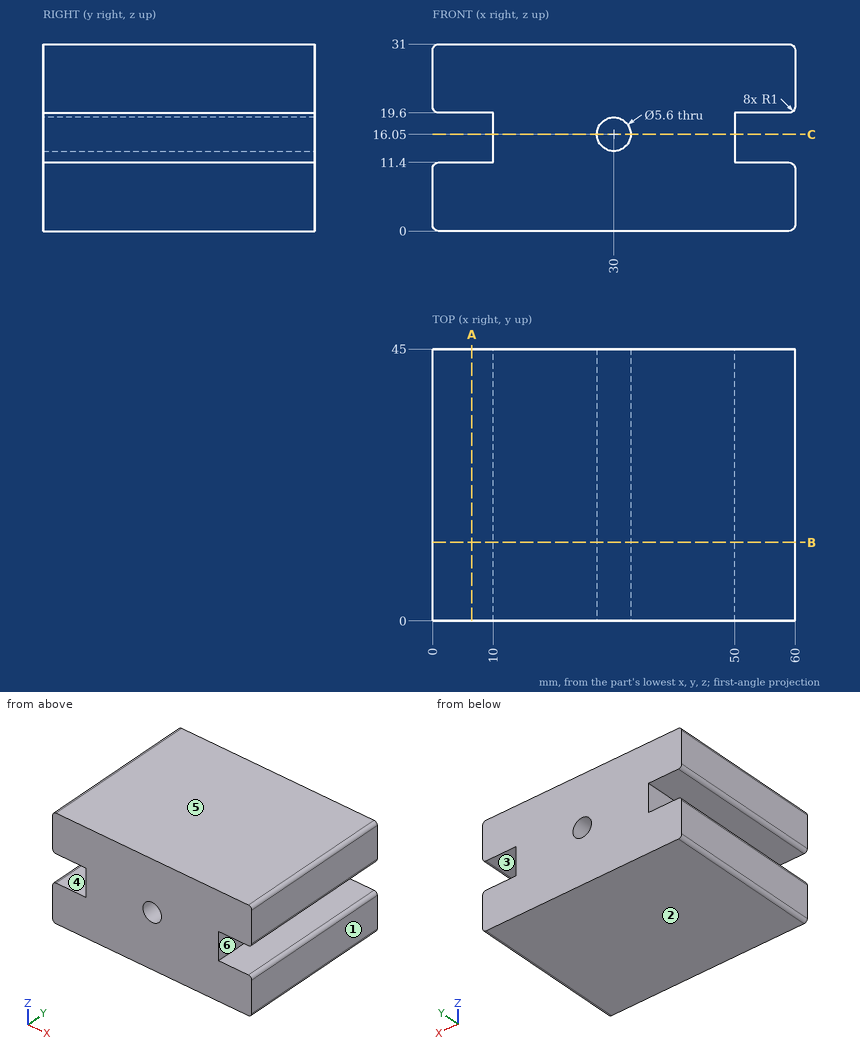
The drawing under review shows one solid part. Ordinate dimensions are in mm from its lowest x, y, z. A direction names the side the tool comes from. Round coordinates to 2 decimals unless told otherwise and drop trailing zeros. Write each loop counter-clockwise with the first axis right and the second up, starting at its lowest first coordinate (ties: lowest second). Pieces come first, ordered by that corner, then holes. Notation, with made-up numbers: (-2.5, 14) - (26.5, 14) arc R27 ccw to (26.5, 31) - close; hole circle Ø2 at (35.5, 24). An arc over 180 degrees is marked (long way). Use a Markdown table: item, result. Add a question column.
1. For the marked faces 4, 5 and 6, list the 3-axis set-ups (+Z, -Z, +X, -X, +Y, -Y) from which the entire face can be reached by the end or side of a thin tool; tool diameter is ignored.
2. We need section C-C (z = 16.05). State the section outline as (x, y) points.
3. We need section A-A (x = 6.5). State the section outline as (y, z) points.
4. We need section B-B (y = 13). State the section outline as (x, z) points, then the cut area to 3 significant figures.
5. Clearance check with a flat-ended pin moving along its axis: pin 1 (6.5 mm diameter, centred on y = 29, z = 16, fed in from +X). State where the tip first meets the part, or that it passes through.
6. Mouldability with a two-part tool opening along Z and no side actions: class the marked faces 1, 2 and 3 as +Z half, -Z half, draft (parallel to the pull), parting line (faces both ways), or undercut.
7. Wall thickness on probe 1 along X at (y, z) = (19.5, 16.05); probe 2 along Z at (x, y) = (30, 27); probe 3 along X at (y, z) = (20, 14): over which ranges is each line inside the solid? List them lowest first.
Output:
| question | item | result |
|---|---|---|
| 1 | face 4 | -X, +Y, -Y |
| 1 | face 5 | +Z, +X, -X, +Y, -Y |
| 1 | face 6 | +X, +Y, -Y |
| 2 | outline | (10, 0) - (27.2, 0) - (27.2, 45) - (10, 45) - close; (32.8, 0) - (50, 0) - (50, 45) - (32.8, 45) - close |
| 3 | outline | (0, 0) - (45, 0) - (45, 11.4) - (0, 11.4) - close; (0, 19.6) - (45, 19.6) - (45, 31) - (0, 31) - close |
| 4 | outline | (0, 1) arc R1 ccw to (1, 0) - (59, 0) arc R1 ccw to (60, 1) - (60, 10.4) arc R1 ccw to (59, 11.4) - (50, 11.4) - (50, 19.6) - (59, 19.6) arc R1 ccw to (60, 20.6) - (60, 30) arc R1 ccw to (59, 31) - (1, 31) arc R1 ccw to (0, 30) - (0, 20.6) arc R1 ccw to (1, 19.6) - (10, 19.6) - (10, 11.4) - (1, 11.4) arc R1 ccw to (0, 10.4) - close; hole circle Ø5.6 at (30, 16.05) |
| 4 | area | 1,670 mm2 |
| 5 | pin 1 | stops at x = 50 |
| 6 | face 1 | draft |
| 6 | face 2 | -Z half |
| 6 | face 3 | undercut |
| 7 | probe 1 | x = 10 to 27.2, 32.8 to 50 |
| 7 | probe 2 | z = 0 to 13.25, 18.85 to 31 |
| 7 | probe 3 | x = 10 to 28.09, 31.91 to 50 |
